CAD build for the part. Positions are in the model's coordinates, mm. Round coordinates to 2 decimals unless told otherwise and drop trailing zeros. Order: outer loops, then holes, each group sorted by start corner. A loop starts at its lowest first (then second) coordinate and runs counter-clockwise, first axis right, second up. Notation, with made-up numbers: (-20.75, 82) -> (6.25, 82) arc R25 ccw to (6.25, 115) -> close; hole circle Ø3 at (2, 34.25). An arc over 180 degrees is marked (long way). Answer as CSV lines item,"result". Start each with the question number.
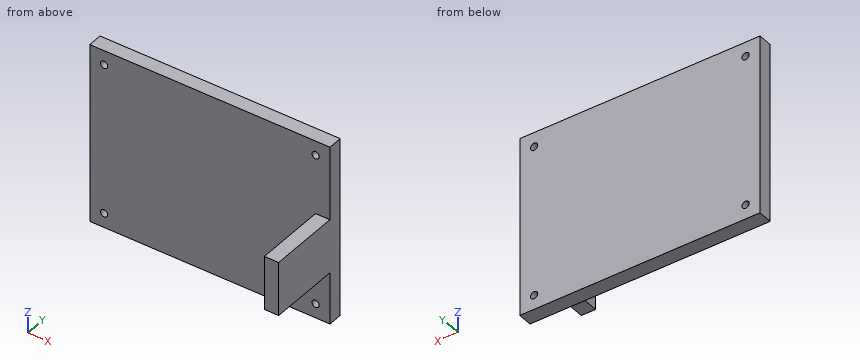
from build123d import *

# Parameters (mm, degrees)
SKETCH1_R           = 0.5
BOSS_EXTRUDE1_DEPTH = 2
SKETCH2_W           = 2
SKETCH2_H           = 7.5
BOSS_EXTRUDE2_DEPTH = 10


with BuildPart() as part:
    # Sketch1 → Boss-Extrude1 (new body)
    # profile 1 of 2: a face of its own
    with BuildSketch(Plane(origin=(0, 9.868787402, 0), x_dir=(1, 0, 0), z_dir=(0, 1, 0))):
        Polygon((40.744370356, 16.373895208), (40.744370356, 8.373895208), (38.744370356, 8.373895208), (38.744370356, 2.373895208), (36.744370356, 2.373895208), (36.744370356, 0.373895208), (11.244370356, 0.373895208), (11.244370356, 2.373895208), (9.244370356, 2.373895208), (9.244370356, 19.373895208), (11.244370356, 19.373895208), (11.244370356, 21.373895208), (36.744370356, 21.373895208), (36.744370356, 19.373895208), (38.744370356, 19.373895208), (38.744370356, 16.373895208), align=None)
    # profile 2 of 2: a face of its own
    with BuildSketch(Plane(origin=(0, 9.868787402, 0), x_dir=(1, 0, 0), z_dir=(0, 1, 0))):
        Polygon((40.744370356, 8.373895208), (38.744370356, 8.373895208), (38.744370356, 2.373895208), (36.744370356, 2.373895208), (36.744370356, 0.373895208), (11.244370356, 0.373895208), (11.244370356, 2.373895208), (9.244370356, 2.373895208), (9.244370356, 19.373895208), (11.244370356, 19.373895208), (11.244370356, 21.373895208), (36.744370356, 21.373895208), (36.744370356, 19.373895208), (38.744370356, 19.373895208), (38.744370356, 16.373895208), (40.744370356, 16.373895208), (40.744370356, 23.373895208), (7.244370356, 23.373895208), (7.244370356, -1.626104792), (40.744370356, -1.626104792), align=None)
        with Locations(Location((9.244370356, 21.373895208, 0), (0, 0, 270))):
            Circle(SKETCH1_R, mode=Mode.SUBTRACT)
        with Locations(Location((38.744370356, 0.373895208, 0), (0, 0, 270))):
            Circle(SKETCH1_R, mode=Mode.SUBTRACT)
        with Locations(Location((38.744370356, 21.373895208, 0), (0, 0, 270))):
            Circle(SKETCH1_R, mode=Mode.SUBTRACT)
        with Locations(Location((9.244370356, 0.373895208, 0), (0, 0, 270))):
            Circle(SKETCH1_R, mode=Mode.SUBTRACT)
    extrude(amount=BOSS_EXTRUDE1_DEPTH)

    # Sketch2 → Boss-Extrude2 (add)
    with BuildSketch(Plane.XZ.offset(-9.868787402)):
        with Locations((39.744370356, -12.373895208)):
            Rectangle(SKETCH2_W, SKETCH2_H)
    extrude(amount=BOSS_EXTRUDE2_DEPTH)


solid = part.part
Item 1: Band-saw the part on A-A, the plane z = -0.5. Give the cut face in (x, y), and give its area (3 significant figures).
Item 2: Band-saw the part on D-D, the plane z = -13.5. Give the cut face in (x, y), and give its area (3 significant figures).
Item 3: Band-saw the part on B-B, the plane x = 26. Give the cut face in (y, z).
Item 4: Band-saw the part on C-C, the plane z = -4.75. Give the cut face in (x, y).
Item 5: Probe line 1 (Z direction, x = 38.5, y = 11); line 2 (Y direction, x = 18.5, z = -12.25); line 3 (X direction, y = 3.25, z = -11.25). List the from-to ranges inside material, lowest first.
Item 6: Pin check, flat tips, straight feed: pin 1 (1 mm diameter, centred on x = 39.5, y = 3, fed in from +Z); pin 2 (4 mm diameter, centred on y = 5, z = -14, fed in from -X); pin 3 (1 mm diameter, centred on x = 39.5, y = 5, fed in from -Z). Stop position of each tip, or through.
Values:
1,outline,"(7.24, 9.87) -> (8.76, 9.87) -> (8.76, 11.87) -> (7.24, 11.87) -> close; (9.73, 9.87) -> (38.26, 9.87) -> (38.26, 11.87) -> (9.73, 11.87) -> close; (39.23, 9.87) -> (40.74, 9.87) -> (40.74, 11.87) -> (39.23, 11.87) -> close"
1,area,"63.1 mm²"
2,outline,"(7.24, 9.87) -> (38.74, 9.87) -> (38.74, -0.13) -> (40.74, -0.13) -> (40.74, 11.87) -> (7.24, 11.87) -> close"
2,area,"87.0 mm²"
3,outline,"(9.87, -23.37) -> (11.87, -23.37) -> (11.87, 1.63) -> (9.87, 1.63) -> close"
4,outline,"(7.24, 9.87) -> (40.74, 9.87) -> (40.74, 11.87) -> (7.24, 11.87) -> close"
5,line 1,"-23.37 to -21.81, -20.94 to -0.81, 0.06 to 1.63"
5,line 2,"9.87 to 11.87"
5,line 3,"38.74 to 40.74"
6,pin 1,"z = -8.62"
6,pin 2,"x = 38.74"
6,pin 3,"z = -16.12"
